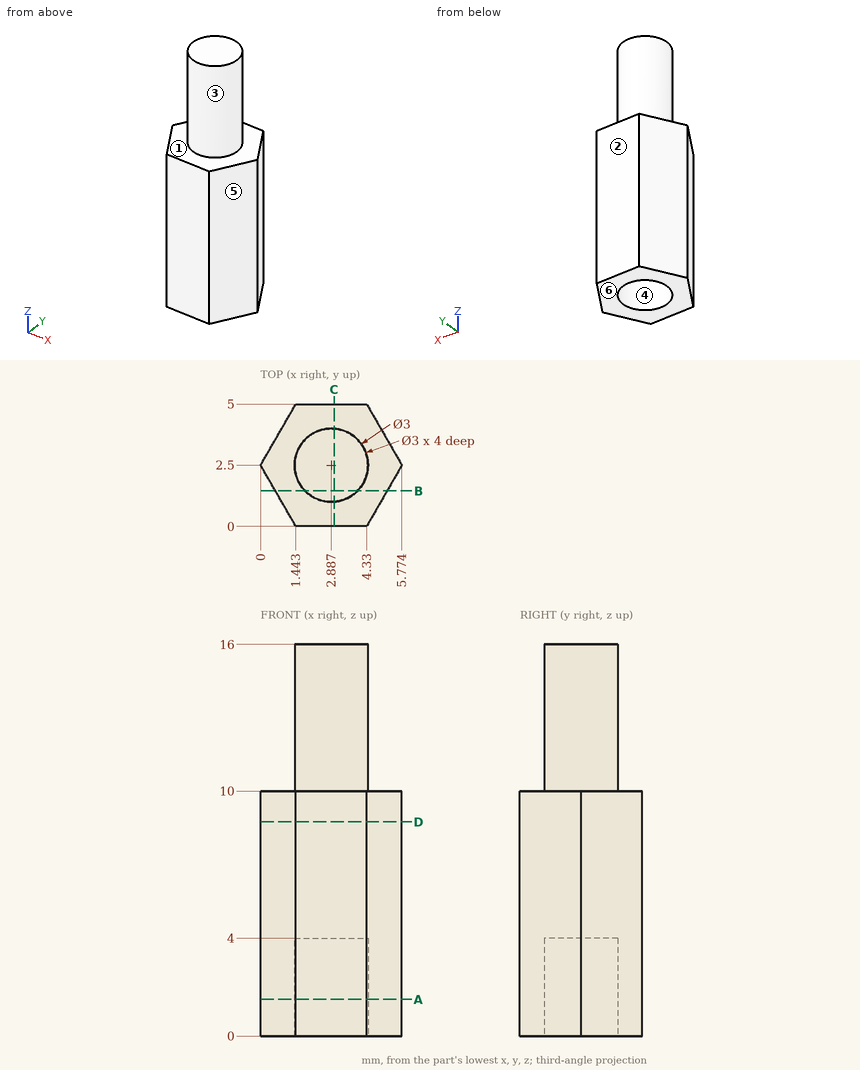
Can you work these out from the drawing? Everything is in mm from the part's minimum corner. A direction names the side the tool comes from. Coordinates: 2 decimals unless noted, no trailing zeros. Loops run counter-clockwise (first coordinate to the right, second up) from the corner with the lowest first, then second, coordinate; pieces in that order, holes last. Notation, with made-up numbers: (-20, -30) -> (39, -30) arc R19 cw to (39, 0) -> close; hole circle Ø2 at (-15, -26). An arc over 180 degrees is marked (long way). Return JSON: item names as keys, results as strings.
1) I need wall thicknesses on line 1 (Z direction, x = 4.1, y = 3.3); line 2 (X direction, y = 2.9, z = 2.25); line 3 (X direction, y = 2.1, z = 13.75). Which ranges of each line are inside material? Lowest first, please. Write a range as from..to.
Results below:
{"line 1": "4..16", "line 2": "0.23..1.44, 4.33..5.54", "line 3": "1.44..4.33"}
2) If we section it at B-B, the plane y = 1.45: Write out the boundary of the cut face in (x, z) (1 decimal), then the cut area to 3 significant figures.
Results below:
{"outline": "(0.6, 0) -> (1.8, 0) -> (1.8, 4) -> (4, 4) -> (4, 0) -> (5.2, 0) -> (5.2, 10) -> (4, 10) -> (4, 16) -> (1.8, 16) -> (1.8, 10) -> (0.6, 10) -> close", "area": "49.9 mm²"}
3) For the marked faces 1 and 2, which set-ups out of +Z, -Z, +X, -X, +Y, -Y let a thin tool reach every point of the face, with its end or its side?
Results below:
{"face 1": "+Z", "face 2": "+Z, -Z, +X, -X, +Y"}
4) If we section it at A-A, the plane z = 1.5: Write out the boundary of the cut face in (x, y), then the cut area to 3 significant figures.
Results below:
{"outline": "(0, 2.5) -> (1.44, 0) -> (4.33, 0) -> (5.77, 2.5) -> (4.33, 5) -> (1.44, 5) -> close; hole circle Ø3 at (2.89, 2.5)", "area": "14.6 mm²"}
5) If we section it at C-C, the plane x = 3: Write out the boundary of the cut face in (y, z) (1 decimal).
Results below:
{"outline": "(0, 0) -> (1, 0) -> (1, 4) -> (4, 4) -> (4, 0) -> (5, 0) -> (5, 10) -> (4, 10) -> (4, 16) -> (1, 16) -> (1, 10) -> (0, 10) -> close"}
6) Will these pins go through, and if not, where does the flat tip stop? pin 1 (1 mm diameter, centred on y = 1.5, z = 8.5, fed in from -X); pin 2 (2.5 mm diameter, centred on x = 2.89, y = 2.5, fed in from -Z); pin 3 (1.5 mm diameter, centred on x = 1.5, z = 13, fed in from -Y).
Results below:
{"pin 1": "x = 0.29", "pin 2": "z = 4", "pin 3": "y = 1.14"}
7) If we section it at D-D, the plane z = 8.75: Write out the boundary of the cut face in (x, y).
Results below:
{"outline": "(0, 2.5) -> (1.44, 0) -> (4.33, 0) -> (5.77, 2.5) -> (4.33, 5) -> (1.44, 5) -> close"}
8) Thinking about a two-plate mould opening in X: for the marked faces 3, 4, 5 and 6, which applies, +X half, -X half, draft (parallel to the pull), parting line (faces both ways), or undercut?
Results below:
{"face 3": "parting line", "face 4": "undercut", "face 5": "+X half", "face 6": "draft"}
